Work out the finished part from the listing and answer in its coordinate system (mm). A direction names the side the tool comes from. Give positions to 0.01 mm unless a question says otherwise; leave off trailing zeros. Loops run counter-clockwise (first coordinate to the right, second up) from the corner with the lowest first, then second, coordinate; pieces in that order, holes last.
```python
from build123d import *

# Parameters (mm, degrees)
F0_R     = 10
F0_R_2   = 9.5
F1_DEPTH = 6
F2_DEPTH = 12
F3_DEPTH = 22


with BuildPart() as f1:
    # F0 (on Top) → F1 (new body)
    with BuildSketch(Plane.XY):
        with BuildLine():
            Line((-95, -17.5), (0, -17.5))
            ThreePointArc((0, -17.5), (17.5, 0), (0, 17.5))
            Line((0, 17.5), (-22, 17.5))
            Line((-22, 17.5), (-22, 12.5))
            Line((-22, 12.5), (-69.5748026423, -5.3779074195))
            Line((-69.5748026423, -5.3779074195), (-99.2765917217, -16.5394006021))
            ThreePointArc((-99.2765917217, -16.5394006021), (-97.1915740894, -17.2568951522), (-95, -17.5))
        make_face()
        Circle(F0_R, mode=Mode.SUBTRACT)
        with BuildLine():
            Line((-22, 12.5), (-22, 17.5))
            Line((-22, 17.5), (-70, 17.5))
            Line((-70, 17.5), (-80, 67.5))
            Line((-80, 67.5), (-105, 67.5))
            Line((-105, 67.5), (-105, 17.5))
            add(Edge.make_bspline(
                [(-105, 17.5), (-92.1195688134, 17.707814564), (-69.750044995, 17.565080001), (-70.398492672, 3.779775432), (-69.5748026423, -2.8830476028)],
                knots=[0, 0, 0, 0, 0.5805224933, 1, 1, 1, 1], degree=3))
            Line((-69.5748026423, -2.8830476028), (-69.5748026423, -5.3779074195))
            Line((-69.5748026423, -5.3779074195), (-22, 12.5))
        make_face()
        with BuildLine():
            ThreePointArc((-105, -7.5), (-103.4488436255, -12.8494898253), (-99.2765917217, -16.5394006021))
            Line((-99.2765917217, -16.5394006021), (-69.5748026423, -5.3779074195))
            Line((-69.5748026423, -5.3779074195), (-69.5748026423, -2.8830476028))
            add(Edge.make_bspline(
                [(-105, 17.5), (-92.1195688134, 17.707814564), (-69.750044995, 17.565080001), (-70.398492672, 3.779775432), (-69.5748026423, -2.8830476028)],
                knots=[0, 0, 0, 0, 0.5805224933, 1, 1, 1, 1], degree=3))
            Line((-105, 17.5), (-105, -7.5))
        make_face()
        with Locations((-85, 0)):
            Circle(F0_R_2, mode=Mode.SUBTRACT)
        with BuildLine():
            Line((-105, 67.5), (-80, 67.5))
            Line((-80, 67.5), (-85.0721864729, 69.5288745892))
            ThreePointArc((-85.0721864729, 69.5288745892), (-92.5, 70.9593407715), (-99.9278135271, 69.5288745892))
            Line((-99.9278135271, 69.5288745892), (-105, 67.5))
        make_face()
    extrude(amount=F1_DEPTH)

    # F0 (on Top) → F2 (join)
    with BuildSketch(Plane.XY):
        with BuildLine():
            ThreePointArc((-105, -7.5), (-103.4488436255, -12.8494898253), (-99.2765917217, -16.5394006021))
            Line((-99.2765917217, -16.5394006021), (-69.5748026423, -5.3779074195))
            Line((-69.5748026423, -5.3779074195), (-69.5748026423, -2.8830476028))
            add(Edge.make_bspline(
                [(-105, 17.5), (-92.1195688134, 17.707814564), (-69.750044995, 17.565080001), (-70.398492672, 3.779775432), (-69.5748026423, -2.8830476028)],
                knots=[0, 0, 0, 0, 0.5805224933, 1, 1, 1, 1], degree=3))
            Line((-105, 17.5), (-105, -7.5))
        make_face()
        with Locations((-85, 0)):
            Circle(F0_R_2, mode=Mode.SUBTRACT)
        with BuildLine():
            Line((-22, 12.5), (-22, 17.5))
            Line((-22, 17.5), (-70, 17.5))
            Line((-70, 17.5), (-80, 67.5))
            Line((-80, 67.5), (-105, 67.5))
            Line((-105, 67.5), (-105, 17.5))
            add(Edge.make_bspline(
                [(-105, 17.5), (-92.1195688134, 17.707814564), (-69.750044995, 17.565080001), (-70.398492672, 3.779775432), (-69.5748026423, -2.8830476028)],
                knots=[0, 0, 0, 0, 0.5805224933, 1, 1, 1, 1], degree=3))
            Line((-69.5748026423, -2.8830476028), (-69.5748026423, -5.3779074195))
            Line((-69.5748026423, -5.3779074195), (-22, 12.5))
        make_face()
        with BuildLine():
            Line((-105, 67.5), (-80, 67.5))
            Line((-80, 67.5), (-85.0721864729, 69.5288745892))
            ThreePointArc((-85.0721864729, 69.5288745892), (-92.5, 70.9593407715), (-99.9278135271, 69.5288745892))
            Line((-99.9278135271, 69.5288745892), (-105, 67.5))
        make_face()
    extrude(amount=F2_DEPTH)

    # F0 (on Top) → F3 (join)
    with BuildSketch(Plane.XY):
        with BuildLine():
            Line((-22, 12.5), (-22, 17.5))
            Line((-22, 17.5), (-70, 17.5))
            Line((-70, 17.5), (-80, 67.5))
            Line((-80, 67.5), (-105, 67.5))
            Line((-105, 67.5), (-105, 17.5))
            add(Edge.make_bspline(
                [(-105, 17.5), (-92.1195688134, 17.707814564), (-69.750044995, 17.565080001), (-70.398492672, 3.779775432), (-69.5748026423, -2.8830476028)],
                knots=[0, 0, 0, 0, 0.5805224933, 1, 1, 1, 1], degree=3))
            Line((-69.5748026423, -2.8830476028), (-69.5748026423, -5.3779074195))
            Line((-69.5748026423, -5.3779074195), (-22, 12.5))
        make_face()
        with BuildLine():
            Line((-105, 67.5), (-80, 67.5))
            Line((-80, 67.5), (-85.0721864729, 69.5288745892))
            ThreePointArc((-85.0721864729, 69.5288745892), (-92.5, 70.9593407715), (-99.9278135271, 69.5288745892))
            Line((-99.9278135271, 69.5288745892), (-105, 67.5))
        make_face()
    extrude(amount=F3_DEPTH)

    # F4: F1 across face


with BuildPart() as f1_1:
    add(f1.part)
    add(f1.part.mirror(Plane(origin=(-78.1474366436, 31.848252571, 22), x_dir=(1, 0, 0), z_dir=(0, 0, 1))))


solid = f1_1.part
```
Q1. Section C-C on y = 64.5 is taken. Give the vertices of the cut face in (x, z).
Q2. Section B-B on x = -28.5 is taken. Give the vertices of the cut face in (y, z), plus the area to 3 significant figures.
Q3. Section A-A on x = 6.5 is taken. Give the vertices of the cut face in (y, z).
Q4. Which of the six approach directions +Z, -Z, +X, -X, +Y, -Y give full straight-line access (tool end or side, diameter ignored) to faces 5 (the face through (-69.575, -4, 22)), 6 (the face through (-2.17, -9.76, 2.96)), 7 (the face through (-29, -4, 6)), 8 (the face through (-22, 15, 22)), 9 (the face through (-42, 17.5, 22))?
Q5. Given pin 1 (13 mm diameter, centred on x = -50.5, z = 20, fed in from +Y); pin 2 (5.5 mm diameter, centred on y = 15.5, z = 29.5, fed in from +X); pin 3 (10 mm diameter, centred on y = 27, z = 38.5, fed in from +X), each flat-ended and moving along its own axis, determine where each tip first touches the part or whether it passes through.
Q6. Consider line 1 along Z through (x, y) = (-38.5, 0); line 2 along Y through (x, z) = (-85, 3); line 3 along Z through (x, y) = (-98.5, -8). Determine where each line is inside the solid, lowest interval first.
Q7. Section D-D on y = 4.5 is taken. State how many separate pieces and enclosed holes the cut face has, plus the area to 3 significant figures.
Q8. Determine the mould class of faces 1 (the face through (-92.39, 70.96, 22.31)), 2 (the face through (-2.17, -9.76, 41.04)), 3 (the face through (-48, -17.5, 41)), 4 (the face through (-52.6, 1, 22.2)) for opening direction X: +X half, -X half, draft (parallel to the pull), parting line (faces both ways), or undercut.
Check result:
1. outline: (-105, 0) - (-79.4, 0) - (-79.4, 44) - (-105, 44) - close
2. outline: (-17.5, 0) - (17.5, 0) - (17.5, 44) - (-17.5, 44) - (-17.5, 38) - (10.06, 38) - (10.06, 6) - (-17.5, 6) - close
2. area: 658 mm2
3. outline: (-16.25, 0) - (-7.6, 0) - (-7.6, 6) - (-16.25, 6) - close; (-16.25, 38) - (-7.6, 38) - (-7.6, 44) - (-16.25, 44) - close; (7.6, 0) - (16.25, 0) - (16.25, 6) - (7.6, 6) - close; (7.6, 38) - (16.25, 38) - (16.25, 44) - (7.6, 44) - close
4. face 5: -X, -Y
4. face 6: +Z, -Z
4. face 7: +X, -Y
4. face 8: +X, +Y, -Y
4. face 9: +Z, -Z, +X, +Y
5. pin 1: stops at y = 17.5
5. pin 2: stops at x = -22
5. pin 3: stops at x = -70.9
6. line 1: z = 0 to 6, 38 to 44
6. line 2: y = -17.5 to -9.5, 9.5 to 69.5
6. line 3: z = 0 to 12, 32 to 44
7. separate pieces: 5
7. enclosed holes: 0
7. area: 2,130 mm2
8. face 1: parting line
8. face 2: undercut
8. face 3: draft
8. face 4: +X half
